Read the model definition and answer for the solid it produces. Units are mm, in the model's axes. A direction names the side the tool comes from. Give positions to 0.01 mm unless a question says otherwise; leave off trailing zeros. Loops run counter-clockwise (first coordinate to the right, second up) from the corner with the lowest first, then second, coordinate; pieces in that order, holes last. Notation, with made-up numbers: (-14.75, 43.5) - (37.25, 43.5) arc R22 ccw to (37.25, 68.5) - close; hole circle Ø1 at (10, 8). An arc over 180 degrees is marked (long way). Write item = value, one per line.
Autodesk Inventor part; units mm, degrees
ref_plane "YZ Plane" through (0, 0, 0) normal (1, 0, 0) x (0, 1, 0)
ref_plane "XZ Plane" through (0, 0, 0) normal (0, 1, 0) x (-1, 0, 0)
ref_plane "XY Plane" through (0, 0, 0) normal (0, 0, 1) x (1, 0, 0)
sketch "Sketch1" plane through (0, 0, 0) normal (0, 1, 0) x (-1, 0, 0)
  circle A0 centre (0, 0) radius 18
  dimension "d1" = 36
extrude "Extrusion1" add sketch "Sketch1" along normal blind 2
sketch "Sketch2" plane through (0, 2, 0) normal (0, 1, 0) x (1, 0, 0)
  circle A0 centre (0, 0) radius 17
  dimension "d4" = 34
extrude "Extrusion2" cut sketch "Sketch2" against normal blind 1.5
ref_plane "Work Plane1" through (-9.8347, 0.5, -3.688) normal (-1, 0, 0) x (0, 0, 1)
sketch "Sketch5" plane through (-9.8347, 0.5, -3.688) normal (-1, 0, 0) x (0, 0, 1)
  point P0 (3.688, -0.5)
ref_plane "Work Plane4" through (-9.8347, 0.5, -3.688) normal (-1, 0, 0) x (0, 0, 1)
sketch "Sketch6" plane through (-9.8347, 0.5, -3.688) normal (-1, 0, 0) x (0, 0, 1)
  line L0 (-13.312, 0) -> (20.688, 0)
  line L1 (21.688, 1.5) -> (-14.312, 1.5)
  line L2 (-1.5361, 0) -> (9.81, 0)
  line L3 (9.81, 0) -> (9.81, 1.5)
  line L4 (9.81, 1.5) -> (-1.5361, 1.5)
  line L5 (-1.5361, 1.5) -> (-1.5361, 0)
  point P0 (3.688, -0.5)
extrude "Extrusion4" cut sketch "Sketch6" along normal blind 15
sketch "Sketch8" plane through (0, 2, 0) normal (0, 1, 0) x (1, 0, 0)
  arc A0 (-16.9269, -6.122) -> (-17.2252, 5.2241) centre (0, 0) ccw
  line L0 (-15.8594, -6.122) -> (-16.9269, -6.122)
  line L1 (-16.9269, -6.122) -> (-15.8594, -6.122)
  arc A1 (-15.8594, -6.122) -> (-16.1774, 5.2241) centre (0, 0) ccw
  arc A2 (-15.8594, -6.122) -> (-16.1774, 5.2241) centre (0, 0) ccw
  arc A3 (-16.9269, -6.122) -> (-17.2252, 5.2241) centre (0, 0) ccw
  arc A4 (-17.2252, 5.2241) -> (-16.9269, -6.122) centre (0, 0) ccw
  line L2 (-16.1774, 5.2241) -> (-17.2252, 5.2241)
  line L3 (-17.2252, 5.2241) -> (-16.1774, 5.2241)
extrude "Extrusion5" add sketch "Sketch8" along normal blind 2.5 contours L0 A1 L2 A0
sketch "Sketch9" plane through (0, 0.5, 0) normal (0, 1, 0) x (1, 0, 0)
  circle A0 centre (0, 0) radius 1.3727
extrude "Extrusion6" add sketch "Sketch9" along normal blind 6
properties part number "watchChargerBottom"
1) A tool of negligible diameter and unlimited length cuts with its end or side. For faces 1 (the face through (-0.3, 3.46, -1.34)), 2 (the face through (-16.4, 2.5, 6.122)), 3 (the face through (0, 6.5, 0)), from which of +Z, -Z, +X, -X, +Y, -Y can it reach the whole face along a straight path? Write none if from no direction.
Output:
face_1 = +Y
face_2 = -X, +Y
face_3 = +Z, -Z, +X, -X, +Y
2) Each of these flat-tipped pins is pushed along its axis until it touches: P1, Ø10.5, axis at x = -3, z = -1, coming from the +Y side; P2, Ø1, axis at x = 5, y = 1.5, coming from the -Z side; P3, Ø5, axis at x = -6.5, z = 1, coming from the +Y side; P4, Ø3, axis at y = 5.5, z = 5.5, coming from the -X side. Where does it stop, or does it pass through?
Output:
P1 = 6.5
P2 = -17.43
P3 = 0.5
P4 = -16.93
3) A cutting plane is placed at D-D on y = 5.25. Determine the outline of the cut face in (x, z).
Output:
outline = circle Ø2.75 at (0, 0)
4) Find the intervals of material crossed by probe 1 along Z at (x, y) = (0, 3.8); probe 2 along X at (y, z) = (1.35, 0); probe 3 along Y at (x, z) = (-3, 3), in increasing order.
Output:
probe_1 = -18 to -17, -1.37 to 1.37, 17 to 18
probe_2 = -1.37 to 1.37, 17 to 18
probe_3 = 0 to 0.5
5) A cutting plane is placed at C-C on y = 1. Determine the outline of the cut face in (x, z).
Output:
outline = (-17.23, -5.22) arc R18 ccw (long way) to (-16.93, 6.12) - (-15.86, 6.12) arc R17 cw (long way) to (-16.18, -5.22) - close; circle Ø2.75 at (0, 0)
